Source: CAD feature listing. Evaluate the final solid. Frame: model axes, mm. Face numbers are marked on the shaded views. A direction names the side the tool comes from. Round coordinates to 2 decimals unless told otherwise and drop trailing zeros. Loops run counter-clockwise (first coordinate to the right, second up) from the corner with the lowest first, then second, coordinate; pieces in that order, holes last. Notation, with made-up numbers: (3.5, 69.25) - (61.5, 69.25) arc R21 cw to (61.5, 90.25) - close; hole circle Ø3 at (43, -39.5). An arc over 180 degrees is marked (long way). One line per question, with ' | ' between items. Start each with the question number.
1. Access query for the marked faces 1 and 2. Directions: +Z, -Z, +X, -X, +Y, -Y. A direction counts if a zero-diameter tool reaches every point of the face in a straight line with its end or side. Return the directions, or none.
2. Cut plane B-B (x = 94.5). Return loops of the section in (y, z), then the cut area to 3 significant figures.
3. Ray query, line 1 (Z direction, x = 103, y = 2.5); line 2 (Z direction, x = 102.5, y = 22.5); line 3 (Y direction, x = 79, z = 4). Return the intervals inside material, ascending.
4. Cut plane C-C (z = 10.5). Return loops of the section in (x, y), then the cut area to 3 significant figures.
5. Pin query (flat end, axial travel): pin 1 (1.5 mm diameter, centred on y = 3, z = 16.5, fed in from +X); pin 2 (1.5 mm diameter, centred on x = 100.5, z = 10.5, fed in from +Y); pin 3 (6 mm diameter, centred on y = 4, z = 5.5, fed in from +X). Return the tip coordinate at first contact, or that it passes through.
6. Cut plane A-A (z = 14.5). Return loops of the section in (x, y).
7. Cut plane D-D (y = 7.25). Return loops of the section in (x, z).
Autodesk Inventor part; units mm, degrees
ref_plane "YZ Plane" through (0, 0, 0) normal (1, 0, 0) x (0, 1, 0)
ref_plane "XZ Plane" through (0, 0, 0) normal (0, 1, 0) x (-1, 0, 0)
ref_plane "XY Plane" through (0, 0, 0) normal (0, 0, 1) x (1, 0, 0)
sketch "Sketch1" plane through (0, 0, 0) normal (0, 0, 1) x (1, 0, 0)
  arc A0 (75, 0) -> (72.4444, 19.4114) centre (0, 0) ccw
  arc A1 (105, 0) -> (101.4222, 27.176) centre (0, 0) ccw
  line L0 (105, 0) -> (75, 0)
  line L1 (72.4444, 19.4114) -> (101.4222, 27.176)
  line L2 (75, 0) -> (0, 0)
  line L3 (0, 0) -> (72.4444, 19.4114)
  circle A2 centre (78.2518, 16.6329) radius 1.25
  circle A3 centre (79.8904, 4.1869) radius 1.25
  circle A4 centre (97.8148, 20.7912) radius 1.25
  circle A5 centre (99.863, 5.2336) radius 1.25
  line L4 (0, 0) -> (78.2518, 16.6329)
  line L5 (78.2518, 16.6329) -> (97.8148, 20.7912)
  line L6 (99.863, 5.2336) -> (79.8904, 4.1869)
  line L7 (79.8904, 4.1869) -> (0, 0)
  dimension "d0" = 20
  dimension "d1" = 15
  dimension "d2" = 3
  dimension "d3" = 3
  dimension "d4" = 2.5
  dimension "d5" = 80
  dimension "d6" = 75
  dimension "d7" = 105
  dimension "d8" = 80
  dimension "d9" = 20
extrude "Extrusion1" add sketch "Sketch1" along normal blind 30 contours A0 L1 A1 L0
ref_plane "Work Plane1" through (0, 0, 15) normal (0, 0, 1) x (1, 0, 0)
sketch "Sketch2" plane through (0, 0, 15) normal (0, 0, 1) x (1, 0, 0)
  line L0 (75, 0) -> (105, 0)
  line L1 (75, 0) -> (0, 0)
  line L2 (0, 0) -> (189.2794, -3.3039)
  line L3 (84.9871, -1.4835) -> (85.214, 11.5165)
  line L4 (85.214, 11.5165) -> (105.2109, 11.1675)
  line L5 (105.2109, 11.1675) -> (104.984, -1.8325)
  dimension "d12" = 13
  dimension "d13" = 1
  dimension "d14" = 85
  dimension "d15" = 105
extrude "Extrusion2" cut sketch "Sketch2" along normal mid plane 12 contours L3 L4 L5 L2
sketch "Sketch3" plane through (104.4029, 11.1816, 9) normal (-0.0174524, -0.9998477, 0) x (0.9998477, -0.0174524, 0)
  arc A0 (-5, 4.3) -> (-5, 7.7) centre (-5, 6) ccw
  arc A1 (-7, 7.7) -> (-7, 4.3) centre (-7, 6) ccw
  line L0 (-7, 7.7) -> (-5, 7.7)
  line L1 (-5, 4.3) -> (-7, 4.3)
  line L2 (-19.1919, 12) -> (0.7921, 12)
  line L3 (0, 12) -> (0, 0)
  point P0 (-104.1919, -9)
  dimension "d19" = 3.4
  dimension "d20" = 6
  dimension "d21" = 5
  dimension "d22" = 2
extrude "Extrusion3" cut sketch "Sketch3" against normal blind 20
pattern_linear "Rectangular Pattern1" count 2 spacing 7.5 along (-0.9998477, 0.0174524, 0) of "Extrusion3"
ref_plane "Work Plane2" through (104.6822, 27.1792, 9) normal (-0.0174524, -0.9998477, 0) x (0.9998477, -0.0174524, 0)
sketch "Sketch5" plane through (104.6822, 27.1792, 9) normal (-0.0174524, -0.9998477, 0) x (0.9998477, -0.0174524, 0)
  line L0 (-19.0973, 2.5) -> (0.9027, 2.5)
  line L1 (0.9027, 2.5) -> (0.9027, 9.5)
  line L2 (0.9027, 9.5) -> (-19.0973, 9.5)
  line L3 (-19.0973, 9.5) -> (-19.0973, 2.5)
  line L4 (-3.2594, 21) -> (-32.0973, 21)
  line L5 (-32.0973, -9) -> (-32.0973, 21)
  point P0 (-104.1919, -9)
  point P1 (-19.0973, 6)
  dimension "d29" = 7
  dimension "d30" = 15
  dimension "d31" = 13
  dimension "d32" = 20
extrude "Extrusion4" cut sketch "Sketch5" along normal blind 5
properties part number "load_cell_mounting_block2"
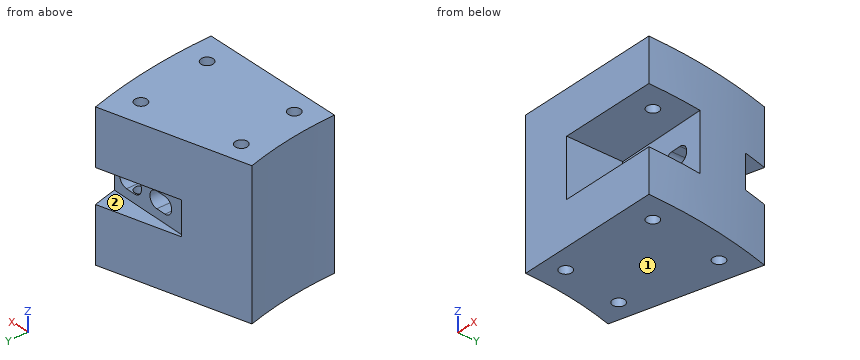
Answers follow:
1) face 1: -Z, +X, -X, +Y, -Y | face 2: +X, +Y
2) outline: (0, 0) - (25.32, 0) - (25.32, 11.5) - (22.35, 11.5) - (22.35, 18.5) - (25.32, 18.5) - (25.32, 30) - (0, 30) - (0, 21) - (11.35, 21) - (11.35, 9) - (0, 9) - close | area: 603 mm2
3) line 1: z = 0 to 9, 21 to 30 | line 2: z = 0 to 11.5, 18.5 to 30 | line 3: y = 0 to 3.31, 5.06 to 15.63, 17.63 to 21.17
4) outline: (72.44, 19.41) arc R75 cw to (75, 0) - (85.01, 0) - (85.21, 11.52) - (104.4, 11.18) arc R105 ccw to (101.42, 27.18) - close; hole circle Ø2.5 at (78.25, 16.63); hole circle Ø2.5 at (79.89, 4.19); hole circle Ø2.5 at (97.81, 20.79) | area: 469 mm2
5) pin 1: stops at x = 85.08 | pin 2: stops at y = 27.13 | pin 3: stops at x = 105
6) outline: (72.44, 19.41) arc R75 cw to (75, 0) - (85.01, 0) - (85.21, 11.52) - (88.28, 11.46) - (88.47, 22.46) - (85.5, 22.51) - (85.51, 22.91) - close; (93.53, 11.37) - (95.78, 11.33) - (95.97, 22.33) - (93.72, 22.37) - close; (101.03, 11.24) - (104.4, 11.18) arc R105 ccw to (102.62, 22.21) - (101.22, 22.24) - close; hole circle Ø2.5 at (78.25, 16.63); hole circle Ø2.5 at (79.89, 4.19)
7) outline: (74.65, 0) - (104.75, 0) - (104.75, 9) - (85.14, 9) - (85.14, 21) - (104.75, 21) - (104.75, 30) - (74.65, 30) - close
